Could you check a few things on this model? Use its own coordinates, in mm. A direction names the side the tool comes from. Give positions to 0.01 mm unless a question says otherwise; leave off trailing zeros. Order: outer loops, then holes, each group sorted by start corner. A loop starts at its lowest first (then second) coordinate and runs counter-clockwise, first axis right, second up. Notation, with made-up numbers: M 46,74.5 L 101,74.5 A15 cw 101,97.5 Z; hole C -10,33 d10. An arc over 180 degrees is marked long. Return JSON: item names as keys, results as strings. Group by question number.
```python
from build123d import *

# Parameters (mm, degrees)
F0_R     = 6.35
F1_DEPTH = 262.636
F0_R_2   = 12.7
F2_DEPTH = 20.574


with BuildPart() as f1:
    # F0 (on Top) → F1 (new body)
    with BuildSketch(Plane.XY):
        Circle(F0_R)
    extrude(amount=F1_DEPTH)

    # F0 (on Top) → F2 (join)
    with BuildSketch(Plane.XY):
        Circle(F0_R_2)
        Circle(F0_R, mode=Mode.SUBTRACT)
        Circle(F0_R)
    extrude(amount=-F2_DEPTH)

    # F3 (on Front) → F4 (revolve, cut)
    with BuildSketch(Plane.XZ):
        with BuildLine():
            Line((7.073207, -20.581745), (7.073207, -25.931608))
            Line((7.073207, -25.931608), (17.550027, -25.931608))
            Line((17.550027, -25.931608), (17.550027, 2.823916))
            Line((17.550027, 2.823916), (7.073207, 2.823916))
            Line((7.073207, 2.823916), (7.073207, 0))
            ThreePointArc((7.073207, 0), (12.381247, -7.393028), (7.073207, -14.786056))
            ThreePointArc((7.073207, -14.786056), (10.592482, -17.6839), (7.073207, -20.581745))
        make_face()
    revolve(axis=Axis((0, 0, -11.275207), (0, 0, -1)), mode=Mode.SUBTRACT)


solid = f1.part
```
1. Imagine slicing it at A-A, the plane z = 145. Please give me the cut outline in (x, y).
2. I need wall thicknesses on L1, parallel to Z at x = 0.25, y = -8.5; L2, parallel to Z at x = 8.25, y = -1.75; L3, parallel to Y at x = -0.75, z = 5.5. Which ranges of each line are inside material? Lowest first, please. Write a range as from..to.
3. Which directions (+Z, -Z, +X, -X, +Y, -Y) give clear straight access to the entire face, cutting with the end or side of a thin tool? Please do faces 1 (the flat face through (0, 0, 262.636)), 2 (the flat face through (-6, 3, 0)).
4. For pin 1 (3 mm diameter, centred on x = 5, z = 194.5, fed in from +Y); pin 2 (2 mm diameter, centred on x = 9, z = 127, fed in from +Y); pin 3 (2 mm diameter, centred on x = -8.5, y = -7, fed in from -Z); pin 4 (3 mm diameter, centred on x = -4, z = 80.5, fed in from -Y), each with a flat end and sliding along its axis, tell me the tip position at first contact or that it passes through.
Values:
{
 "1": {"outline": "C 0,0 d12.7"},
 "2": {"L1": "z = -20.51..-14.86, -14.14..-0.65", "L2": "z = -20.53..-14.84, -14.18..-0.61", "L3": "y = -6.31..6.31"},
 "3": {"face 1": "+Z, +X, -X, +Y, -Y", "face 2": "+Z"},
 "4": {"pin 1": "stops at y = 5.3", "pin 2": "passes through", "pin 3": "stops at z = -19.44", "pin 4": "stops at y = -5.84"}
}
